Verification items for the finished model (mm, model axes). A direction names the side the tool comes from. Give positions to 0.01 mm unless a question says otherwise; leave off trailing zeros. Loops run counter-clockwise (first coordinate to the right, second up) from the corner with the lowest first, then second, coordinate; pieces in that order, holes last. Notation, with made-up numbers: (68, 62.25) - (78, 62.25) arc R19 cw to (78, 81.25) - close; hole circle Ø10 at (24.5, 49.5). An arc over 180 degrees is marked (long way). Put each result on its own line as item: value. Start each with the question number.
Autodesk Inventor part; units mm, degrees
ref_plane "YZ Plane" through (0, 0, 0) normal (1, 0, 0) x (0, 1, 0)
ref_plane "XZ Plane" through (0, 0, 0) normal (0, 1, 0) x (-1, 0, 0)
ref_plane "XY Plane" through (0, 0, 0) normal (0, 0, 1) x (1, 0, 0)
sketch "Sketch1" plane through (0, 0, 0) normal (0, 0, 1) x (1, 0, 0)
  line L0 (-99, 12) -> (99, 12)
  line L1 (99, 12) -> (99, -12)
  line L2 (99, -12) -> (-99, -12)
  line L3 (-99, -12) -> (-99, 12)
  line L4 (-99, 12) -> (99, -12) construction
  line L5 (99, 12) -> (-99, -12) construction
  point P0 (0, 0)
  dimension "d0" = 24
  dimension "d1" = 198
extrude "Extrusion1" add sketch "Sketch1" along normal blind 30
sketch "Sketch2" plane through (-99, 12, 0) normal (0, 1, 0) x (1, 0, 0)
  line L0 (0, 0) -> (0, -30)
  line L1 (0, -15) -> (198, -15)
  line L2 (198, -15) -> (198, 9)
  line L3 (198, 9) -> (0, 9)
  line L4 (0, 9) -> (0, -15)
  line L5 (198, 0) -> (198, -30)
  line L6 (198, 0) -> (0, 0)
  point P0 (99, 0)
  dimension "d4" = 9
extrude "Extrusion2" add sketch "Sketch2" along normal blind 50
fillet "Fillet1" radius 10 1 edges at (0, 62, 15)
sketch "Sketch3" plane through (-99, 62, 0) normal (0, 1, 0) x (1, 0, 0)
  line L0 (0, -30) -> (198, -30)
  line L1 (198, 0) -> (198, -30)
  line L2 (155, -16.5) -> (198, -16.5) construction
  line L3 (43, -16.5) -> (0, -16.5) construction
  line L4 (0, -15) -> (0, -30)
  point P0 (99, 0)
  dimension "d17" = 13.5
  dimension "d19" = 13.5
  dimension "d21" = 112
hole "Hole1" at (56, 62, 16.5) at (-56, 62, 16.5) direction (0, -1, 0) diameter 8.2 end through all counterbore diameter 20 counterbore depth 50
sketch "Sketch4" plane through (-99, -12, 0) normal (0, -1, 0) x (1, 0, 0)
  line L0 (198, 16.5) -> (0, 16.5) construction
  line L1 (0, 0) -> (0, 30)
  line L2 (198, 0) -> (198, 30)
  line L3 (0, 30) -> (198, 30)
  circle A0 centre (155, 16.5) radius 4.1
  circle A1 centre (155, 16.5) radius 4.1
  line L4 (10.5, 25) -> (187.5, 25)
  line L5 (10.5, 8) -> (187.5, 8)
  arc A2 (187.5, 8) -> (187.5, 25) centre (187.5, 16.5) ccw
  arc A3 (10.5, 25) -> (10.5, 8) centre (10.5, 16.5) ccw
  line L6 (10.5, 16.5) -> (0, 16.5)
  line L7 (187.5, 16.5) -> (198, 16.5)
  point P0 (99, 0)
  point P1 (15, 16.5)
  point P2 (99, 16.5)
  point P3 (127, 16.5)
  point P4 (183, 16.5)
  point P5 (71, 16.5)
  dimension "d23" = 56
  dimension "d24" = 28
  dimension "d26" = 28
  dimension "d27" = 28
  dimension "d28" = 56
  dimension "d37" = 17
  dimension "d38" = 177
extrude "Extrusion3" cut sketch "Sketch4" against normal blind 10 contours A3 L4 A2 L5
sketch "Sketch5" plane through (-99, -2, 0) normal (0, -1, 0) x (1, 0, 0)
  circle A0 centre (43, 16.5) radius 10
  circle A1 centre (43, 16.5) radius 4.1
  circle A2 centre (155, 16.5) radius 10
  circle A3 centre (155, 16.5) radius 4.1
  circle A4 centre (43, 16.5) radius 4.1
  circle A5 centre (155, 16.5) radius 4.1
  point P0 (99, 0)
  dimension "d41" = 20
extrude "Extrusion4" add sketch "Sketch5" along normal blind 10
properties part number "13042026-15"
1) Section check B-B, the plane y = 4.5. Enter the section's corners in (x, z), plus the area to 3 significant figures.
2) Section check D-D, the plane y = 47.5. Enter the section's corners in (x, z), plus the area to 3 significant figures.
3) Depth check by flat-ended pin: P1, Ø10, axis at x = -85, y = 24.5, coming from the +Z side; P2, Ø10, axis at x = -60, y = 44.5, coming from the +Z side; P3, Ø12, axis at x = -37, y = -4.5, coming from the -Z side. Enter the tip coordinate at first touch or a pass-through.
4) Set-up check for faces 5 (the face through (82, 32, 15)), 6 (the face through (-1, 12, -5)), 7 (the face through (55.8, 36.6, 6.5)), 8 (the face through (-79, -2, 17)): record each of +Z, -Z, +X, -X, +Y, -Y from which the full face is reachable in a straight line by a thin tool's end or side.
5) Section check A-A, the plane x = -56. Enter the section's corners in (y, z).
6) Scan lines: line 1 along X through (y, z) = (-9, 16); line 2 along X through (y, z) = (7, 16.5); line 3 along Z through (x, y) = (56, 4). Record each from-to range of solid material in increasing order. Write a range as from..to.
7) Draft check along X on faces 1 (the face through (99, 26, 6)), 2 (the face through (75, -7, 25)), 3 (the face through (-99, 24, 6)), 4 (the face through (-1, -2, 17)). Enter one of: pulls with the +X half, pulls with the -X half, needs draft (parallel to the pull), parting line crosses it, or undercut.
8) Section check C-C, the plane x = 26. Enter the section's corners in (y, z), plus the area to 3 significant figures.
Results are:
1. outline: (-99, 0) - (99, 0) - (99, 30) - (-99, 30) - close; hole circle Ø8.2 at (-56, 16.5); hole circle Ø8.2 at (56, 16.5)
1. area: 5,830 mm2
2. outline: (-99, -9) - (99, -9) - (99, 15) - (65.89, 15) arc R10 cw to (46.11, 15) - (-46.11, 15) arc R10 cw to (-65.89, 15) - (-99, 15) - close
2. area: 4,500 mm2
3. P1: stops at z = 15
3. P2: stops at z = 12.14
3. P3: stops at z = 0
4. face 5: +Z, +X, -X, +Y
4. face 6: -Z, +X, -X, -Y
4. face 7: +Z, +Y
4. face 8: -Y
5. outline: (-12, 0) - (12, 0) - (12, -9) - (62, -9) - (62, 5) arc R10 ccw to (61.89, 6.5) - (12, 6.5) - (12, 12.4) - (-12, 12.4) - close; (-12, 20.6) - (12, 20.6) - (12, 30) - (-12, 30) - close
6. line 1: x = -99..-96.99, -65.99..-60.07, -51.93..-46.01, 46.01..51.93, 60.07..65.99, 96.99..99
6. line 2: x = -99..-60.1, -51.9..51.9, 60.1..99
6. line 3: z = 0..12.4, 20.6..30
7. face 1: pulls with the +X half
7. face 2: undercut
7. face 3: pulls with the -X half
7. face 4: undercut
8. outline: (-12, 0) - (12, 0) - (12, -9) - (62, -9) - (62, 5) arc R10 ccw to (52, 15) - (12, 15) - (12, 30) - (-12, 30) - (-12, 25) - (-2, 25) - (-2, 8) - (-12, 8) - close
8. area: 1,730 mm2
